from build123d import *

# Parameters (mm, degrees)
SKETCH013_R     = 9.5
PAD011_DEPTH    = 32
SKETCH014_R     = 4
POCKET002_DEPTH = 30
SKETCH015_R     = 6
PAD012_DEPTH    = 23


with BuildPart() as part:
    # Sketch013 → Pad011 (new body)
    with BuildSketch(Plane.XZ):
        Circle(SKETCH013_R)
    extrude(amount=PAD011_DEPTH)

    # Sketch014 (on Face2 of Pad011) → Pocket002 (cut)
    with BuildSketch(Plane(origin=(0, 0, 0), x_dir=(1, 0, 0), z_dir=(0, 1, 0))):
        Circle(SKETCH014_R)
    extrude(amount=-POCKET002_DEPTH, mode=Mode.SUBTRACT)

    # Sketch015 (on Face3 of Pocket002) → Pad012 (new body)
    with BuildSketch(Plane.XZ.offset(32)):
        Circle(SKETCH015_R)
    extrude(amount=PAD012_DEPTH)


solid = part.part
Check sheet for the modelled part. Datum: model origin and axes. Units: mm. A direction names the side the tool comes from. Give positions to 0.01 mm unless a question says otherwise; leave off trailing zeros. Write each loop counter-clockwise with the first axis right and the second up, starting at its lowest first coordinate (ties: lowest second). Pieces come first, ordered by that corner, then holes. Notation, with made-up numbers: (60.5, 21) -> (105.5, 21) arc R30 ccw to (105.5, 48) -> close; hole circle Ø3 at (22.5, 88). An arc over 180 degrees is marked (long way). One line per item, written item: value. Start each with the question number.
Item 1: Section check D-D on y = -35. Record the cut outline in (x, z), then the cut area to 3 significant figures.
Item 2: Gauge pin test, flat ends, axial feed: pin 1 (3 mm diameter, centred on y = -15, z = -7, fed in from -X); pin 2 (8 mm diameter, centred on y = -18.5, z = 5.5, fed in from -X); pin 3 (4 mm diameter, centred on x = -6.5, y = -11, fed in from -Z). Record the tip position at first contact, or that the pin passes through.
Item 3: Section check B-B on x = 0. Record the cut outline in (y, z), then the cut area to 3 significant figures.
Item 4: Section check A-A on z = 0. Record the cut outline in (x, y).
Item 5: Section check C-C on y = -15.5. Record the cut outline in (x, z).
Item 6: Tool access check on faces 4 (the flat face through (-0.1, -32, -6.2)), 5 (the flat face through (0, -30, 0)), 6 (the flat face through (0, -55, 0)). Record the directions out of +Z, -Z, +X, -X, +Y, -Y that give a thin tool (end or side, any length) a straight path to the whole face; none if there is none.
Item 7: Draft check along Z on faces 1 (the flat face through (4, 0, -2)), 2 (the cylindrical face through (-6, -43, 0)), 3 (the cylindrical face through (-0.867, -14.79, 3.905)). Enter one of: +Z half, -Z half, draft (parallel to the pull), parting line (faces both ways), or undercut.
Item 8: Material ranges on probe 1 along Z at (x, y) = (0, -21.25); probe 2 along Y at (x, z) = (7, 0.75); probe 3 along X at (y, z) = (-26.5, -3), recorded low to high. Write a range as from..to.
Results list:
1. outline: circle Ø12 at (0, 0)
1. area: 113 mm²
2. pin 1: x = -7.75
2. pin 2: x = -9.38
2. pin 3: z = -8.37
3. outline: (-55, -6) -> (-32, -6) -> (-32, -9.5) -> (0, -9.5) -> (0, -4) -> (-30, -4) -> (-30, 4) -> (0, 4) -> (0, 9.5) -> (-32, 9.5) -> (-32, 6) -> (-55, 6) -> close
3. area: 644 mm²
4. outline: (-9.5, -32) -> (-6, -32) -> (-6, -55) -> (6, -55) -> (6, -32) -> (9.5, -32) -> (9.5, 0) -> (4, 0) -> (4, -30) -> (-4, -30) -> (-4, 0) -> (-9.5, 0) -> close
5. outline: circle Ø19 at (0, 0); hole circle Ø8 at (0, 0)
6. face 4: -Y
6. face 5: +Y
6. face 6: +Z, -Z, +X, -X, -Y
7. face 1: draft
7. face 2: parting line
7. face 3: undercut
8. probe 1: -9.5..-4, 4..9.5
8. probe 2: -32..0
8. probe 3: -9.01..-2.65, 2.65..9.01
